Verification items for the finished model (mm, model axes). A direction names the side the tool comes from. Round coordinates to 2 decimals unless told otherwise and drop trailing zeros. Loops run counter-clockwise (first coordinate to the right, second up) from the corner with the lowest first, then second, coordinate; pieces in that order, holes last. Notation, with made-up numbers: (79.25, 27) -> (117.25, 27) arc R19 cw to (117.25, 35) -> close; hole circle Ø3 at (4.5, 45). An arc over 180 degrees is marked (long way). Use CSV: the item, a comma, the result in double quotes. Start each with the question number.
```python
from build123d import *

# Parameters (mm, degrees)
SKETCH1_W                  = 38
SKETCH1_H                  = 56
BOSS_EXTRUDE1_DEPTH        = 2
SKETCH2_W                  = 5
SKETCH2_H                  = 38.1
SKETCH2_H_2                = 50.8
BOSS_EXTRUDE2_DEPTH        = 2
F_3_2_3_2_DIAMETER_HOLE1_D = 3.2


with BuildPart() as part:
    # Sketch1 → Boss-Extrude1 (new body)
    with BuildSketch(Plane(origin=(0, 0, 0), x_dir=(1, 0, 0), z_dir=(0, 1, 0))):
        Rectangle(SKETCH1_W, SKETCH1_H)
    extrude(amount=BOSS_EXTRUDE1_DEPTH)

    # Sketch2 → Boss-Extrude2 (add)
    with BuildSketch(Plane(origin=(0, 2, 0), x_dir=(1, 0, 0), z_dir=(0, 1, 0))):
        with Locations((-13.5, -6.35)):
            Rectangle(SKETCH2_W, SKETCH2_H)
        with Locations((13.5, 0)):
            Rectangle(SKETCH2_W, SKETCH2_H_2)
    extrude(amount=BOSS_EXTRUDE2_DEPTH)

    # Ø3.2 (3.2) Diameter Hole1 (through all)
    with Locations(Plane(origin=(0, 2, 0), x_dir=(1, 0, 0), z_dir=(0, 1, 0))):
        with Locations((-8, -20), (8, -20), (-8, 20), (8, 20)):
            Hole(F_3_2_3_2_DIAMETER_HOLE1_D / 2)


solid = part.part
```
Q1. Release check for a two-part mould opening along Z. For faces 1 (the face through (0, 1, -28)), 2 (the face through (-7.792, 0.986, 18.414)), 3 (the face through (16, 3, 0)) record: +Z half, -Z half, draft (parallel to the pull), parting line (faces both ways), or undercut.
Q2. Cross-section at A-A (x = -8). Record the boundary of the cut face in (y, z), and give its area (3 significant figures).
Q3. Cross-section at D-D (z = 7.5). Record the boundary of the cut face in (x, y), and give its area (3 significant figures).
Q4. Depth check by flat-ended pin: pin 1 Ø2 at (x, z) = (-8, -5) entering from -Y; pin 2 Ø3 at (x, z) = (-8, -20) entering from +Y; pin 3 Ø1 at (y, z) = (3.5, 9.5) entering from -X; pin 4 Ø0.6 at (y, z) = (2.5, 7.5) entering from +X. Enter the tip coordinate at first touch or a pass-through.
Q5. Cross-section at B-B (y = 1.4). Record the boundary of the cut face in (x, z).
Q6. Thickness scan on L1, parallel to X at y = 0.35, z = 20; L2, parallel to Z at x = 8, y = 1.1; L3, parallel to X at y = 3.25, z = 20.5. Record the ranges inside material, lowest first. Write a range as from..to.
Q7. Tool access check on faces 4 (the face through (-16, 3, 7)), 5 (the face through (-14, 3, -12.7)), 6 (the face through (-11, 3, 7)), 7 (the face through (-14, 3, 25.4)). Record the directions out of +Z, -Z, +X, -X, +Y, -Y that give a thin tool (end or side, any length) a straight path to the whole face; none if there is none.
Q8. Cross-section at C-C (z = -20). Record the boundary of the cut face in (x, y).
Answer list:
1,face 1,"-Z half"
1,face 2,"undercut"
1,face 3,"draft"
2,outline,"(0, -28) -> (2, -28) -> (2, -21.6) -> (0, -21.6) -> close; (0, -18.4) -> (2, -18.4) -> (2, 18.4) -> (0, 18.4) -> close; (0, 21.6) -> (2, 21.6) -> (2, 28) -> (0, 28) -> close"
2,area,"99.2 mm2"
3,outline,"(-19, 0) -> (19, 0) -> (19, 2) -> (16, 2) -> (16, 4) -> (11, 4) -> (11, 2) -> (-11, 2) -> (-11, 4) -> (-16, 4) -> (-16, 2) -> (-19, 2) -> close"
3,area,"96.0 mm2"
4,pin 1,"stops at y = 0"
4,pin 2,"passes through"
4,pin 3,"stops at x = -16"
4,pin 4,"stops at x = 16"
5,outline,"(-19, -28) -> (19, -28) -> (19, 28) -> (-19, 28) -> close; hole circle Ø3.2 at (-8, -20); hole circle Ø3.2 at (-8, 20); hole circle Ø3.2 at (8, -20); hole circle Ø3.2 at (8, 20)"
6,L1,"x = -19..-9.6, -6.4..6.4, 9.6..19"
6,L2,"z = -28..-21.6, -18.4..18.4, 21.6..28"
6,L3,"x = -16..-11, 11..16"
7,face 4,"+Z, -Z, -X, +Y"
7,face 5,"-Z, -X, +Y"
7,face 6,"+Z, -Z, +Y"
7,face 7,"+Z, +X, -X, +Y"
8,outline,"(-19, 0) -> (-9.6, 0) -> (-9.6, 2) -> (-19, 2) -> close; (-6.4, 0) -> (6.4, 0) -> (6.4, 2) -> (-6.4, 2) -> close; (9.6, 0) -> (19, 0) -> (19, 2) -> (16, 2) -> (16, 4) -> (11, 4) -> (11, 2) -> (9.6, 2) -> close"
